The model under review builds one solid part; all positions refer to its coordinate system, in mm. Face numbers are marked on the shaded views. Coordinates: 2 decimals unless noted, no trailing zeros. Order: outer loops, then holes, each group sorted by start corner. A loop starts at its lowest first (then second) coordinate and runs counter-clockwise, first axis right, second up. Notation, with made-up numbers: M 84,46 L 99,46 A36 cw 99,84 Z; hole C 21,-4 d6. An arc over 180 degrees is marked long. Write each question's results on one line, items separated by ' | '.
from build123d import *

# Parameters (mm, degrees)
F0_W     = 16
F0_H     = 2
F1_DEPTH = 30.5
F2_R     = 2.5
F3_W     = 23
F3_H     = 2
F4_DEPTH = 25
F5_SIZE  = 0.5


with BuildPart() as f1:
    # F0 (on Top) → F1 (new body)
    with BuildSketch(Plane.XY):
        Polygon((54.3318165131, 15.8888510838), (-8.6681834869, 15.8888510838), (-8.6681834869, 9.8888510838), (11.3318165131, 9.8888510838), (11.3318165131, 12.8888510838), (34.3318165131, 12.8888510838), (34.3318165131, 9.8888510838), (54.3318165131, 9.8888510838), align=None)
        with Locations((1.3318165131, 12.8888510838)):
            Rectangle(F0_W, F0_H, mode=Mode.SUBTRACT)
        with Locations((44.3318165131, 12.8888510838)):
            Rectangle(F0_W, F0_H, mode=Mode.SUBTRACT)
    extrude(amount=F1_DEPTH)

    # F2
    f2_edges = [f1.edges().sort_by_distance(p)[0] for p in [
        (-8.668183, 9.888851, 15.25),
        (54.331817, 9.888851, 15.25),
    ]]
    fillet(f2_edges, radius=F2_R)

    # F3 (on face) → F4 (cut)
    with BuildSketch(Plane.XZ.offset(-12.8888510838)):
        with Locations((22.8318165131, 1)):
            Rectangle(F3_W, F3_H)
        with Locations((22.8318165131, 29.5)):
            Rectangle(F3_W, F3_H)
    extrude(amount=-F4_DEPTH, mode=Mode.SUBTRACT)

    # F5
    f5_edges = [f1.edges().sort_by_distance(p)[0] for p in [
        (11.331817, 12.888851, 30.5),
        (34.331817, 12.888851, 30.5),
        (34.331817, 12.888851, 0),
        (11.331817, 12.888851, 0),
        (22.831817, 12.888851, 2),
        (22.831817, 12.888851, 28.5),
    ]]
    chamfer(f5_edges, length=F5_SIZE)


solid = f1.part
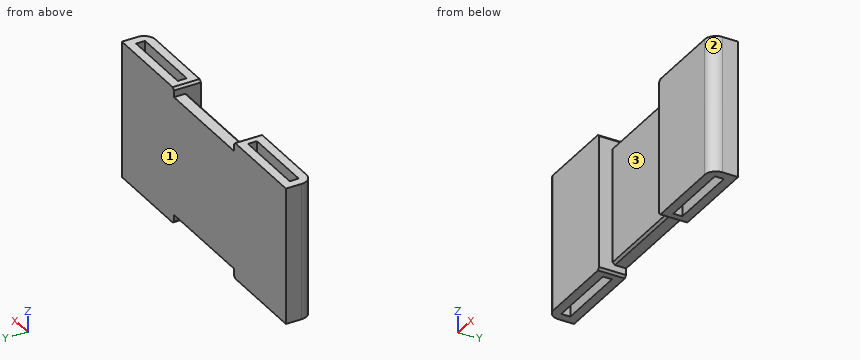
1) Take a section at D-D on x = 26. State the section outline as (y, z) points, plus the area to 4 significant figures.
Solutions:
outline: M 12.89,2.5 L 13.39,2 L 15.89,2 L 15.89,28.5 L 13.39,28.5 L 12.89,28 Z | area: 79.25 mm2
2) To check wall thickness, follow line 1 along X through (y, z) = (12.75, 4.5); line 2 along X through (y, z) = (13.5, 25); line 3 along Y through (x, z) = (-4.5, 20). State the ranges of each line that lie inside material, in increasing order.
Solutions:
line 1: -8.67 to -6.67, 9.33 to 11.33, 34.33 to 36.33, 52.33 to 54.33 | line 2: -8.67 to -6.67, 9.33 to 36.33, 52.33 to 54.33 | line 3: 9.89 to 11.89, 13.89 to 15.89
3) Take a section at C-C on y = 11. State the section outline as (x, z) points.
Solutions:
outline: M -8.25,0 L 10.83,0 L 11.33,0.5 L 11.33,30 L 10.83,30.5 L -8.25,30.5 Z; M 34.33,0.5 L 34.83,0 L 53.91,0 L 53.91,30.5 L 34.83,30.5 L 34.33,30 Z
4) For pin 1 (11.5 mm diameter, centred on x = 21.5, z = 18.5, fed in from -Y); pin 2 (0.8 mm diameter, centred on x = 20, y = 14.5, fed in from -Z); pin 3 (0.8 mm diameter, centred on x = 27.5, y = 14, fed in from +Z), all flat-tipped, find the tip position at first contact; note any pin that passes through.
Solutions:
pin 1: y = 12.89 | pin 2: z = 2 | pin 3: z = 28.5
5) Take a section at A-A on x = 5. State the section outline as (y, z) points.
Solutions:
outline: M 9.89,0 L 11.89,0 L 11.89,30.5 L 9.89,30.5 Z; M 13.89,0 L 15.89,0 L 15.89,30.5 L 13.89,30.5 Z
6) The part is to be moulded in two halves that separate along X. For the marked faces 1, 2 and 3, say which applies: pulls with the +X half, pulls with the -X half, needs draft (parallel to the pull), parting line crosses it, or undercut.
Solutions:
face 1: needs draft | face 2: pulls with the +X half | face 3: undercut
7) Take a section at B-B on z = 23.5. State the section outline as (x, y) points, plus the area to 3 significant figures.
Solutions:
outline: M -8.67,12.39 A2.5 ccw -6.17,9.89 L 11.33,9.89 L 11.33,12.89 L 34.33,12.89 L 34.33,9.89 L 51.83,9.89 A2.5 ccw 54.33,12.39 L 54.33,15.89 L -8.67,15.89 Z; hole M -6.67,11.89 L 9.33,11.89 L 9.33,13.89 L -6.67,13.89 Z; hole M 36.33,11.89 L 52.33,11.89 L 52.33,13.89 L 36.33,13.89 Z | area: 242 mm2
